For this review, take the finished solid that the model builds, in its own axes (mm). Round coordinates to 2 decimals unless told otherwise and drop trailing zeros. Order: outer loops, then holes, each group sorted by start corner. A loop starts at its lowest first (then second) coordinate and runs counter-clockwise, first axis right, second up.
```python
from build123d import *

# Parameters (mm, degrees)
PAD003_DEPTH            = 1.42
POCKET004_DEPTH         = 8.875
POCKET005_DEPTH         = 6.285457
CHAMFER002_SIZE         = 0.5
BODY001_PLACEMENT_ANGLE = 180


with BuildPart() as part:
    # Sketch010 → Pad003 (new body)
    with BuildSketch(Plane.XZ):
        Polygon((-3.142229, 35.5), (3.142229, 35.5), (3.142229, 44.375), (3.142229, 71), (-3.142229, 71), (-3.142229, 44.375), align=None)
    extrude(amount=PAD003_DEPTH)

    # Sketch011 (on Face1 of Pad003) → Pocket004 (cut)
    with BuildSketch(Plane(origin=(0, 0, 35.5), x_dir=(1, 0, 0), z_dir=(0, 0, -1))):
        Polygon((-2.142229, 1.42), (-2.142229, 1), (-7.142229, 1), (-7.142229, 4.921038), align=None)
        Polygon((7.142229, 4.921038), (2.142229, 1.42), (2.142229, 1), (7.142229, 1), align=None)
    extrude(amount=-POCKET004_DEPTH, mode=Mode.SUBTRACT)

    # Sketch012 (on Face9 of Pocket004) → Pocket005 (cut, through all)
    with BuildSketch(Plane(origin=(-3.142229, 0, 0), x_dir=(0, 0, -1), z_dir=(-1, 0, 0))):
        Polygon((-71, 0.19), (-71, 14.02), (-44.375, 1.42), align=None)
    extrude(amount=-POCKET005_DEPTH, mode=Mode.SUBTRACT)

    # Chamfer002
    chamfer002_edges = [part.edges().sort_by_distance(p)[0] for p in [
        (-2.642229, -1, 35.5),
        (-2.142229, -1.21, 35.5),
        (0, -1.42, 35.5),
        (2.142229, -1.21, 35.5),
        (2.642229, -1, 35.5),
        (-3.142229, -0.5, 35.5),
        (3.142229, -0.5, 35.5),
    ]]
    chamfer(chamfer002_edges, length=CHAMFER002_SIZE)


with BuildPart() as part_1:
    # Body001 placement: moved
    add(part.part.moved(Location((0, 25, 32))).rotate(Axis((0, 25, 32), (-1, 0, 0)), BODY001_PLACEMENT_ANGLE))


solid = part_1.part
```
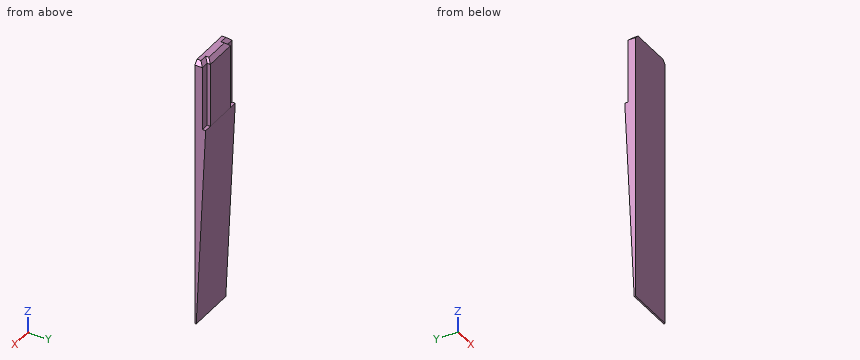
Q1. Take a section at B-B, the plane z = -35. State the section outline as (x, y) points.
Q2. Wall thickness on line 1 (X direction, y = 26.2, z = -10); line 2 (Y direction, x = -0.75, z = -37); line 3 (Y direction, x = 2.25, z = -22): over which ranges is each line inside the solid? List them lowest first.
Q3. Take a section at C-C, the plane z = -13. State the section outline as (x, y) points.
Q4. Clearance check with flat-ended pins moving along their axes: pin 1 (0.5 mm diameter, centred on x = -2.5, z = -7, fed in from +Y); pin 2 (0.5 mm diameter, centred on x = 2.5, y = 26, fed in from +Z); pin 3 (3 mm diameter, centred on x = -0.5, z = -21, fed in from +Y). State where each tip first meets the part, or that it passes through.
Q5. Take a section at A-A, the plane x = 0. State the section outline as (y, z) points (3 decimals), plus the area to 3 significant figures.
Working result:
1. outline: (-3.14, 25) - (3.14, 25) - (3.14, 25.37) - (-3.14, 25.37) - close
2. line 1: x = -2.14 to 2.14
2. line 2: y = 25 to 25.28
2. line 3: y = 25 to 25.98
3. outline: (-3.14, 25) - (3.14, 25) - (3.14, 26.39) - (-3.14, 26.39) - close
4. pin 1: stops at y = 26
4. pin 2: stops at z = -3.75
4. pin 3: stops at y = 26.09
5. outline: (25, -39) - (25.19, -39) - (26.42, -12.375) - (26.42, -4) - (25.92, -3.5) - (25, -3.5) - close
5. area: 33.9 mm2
